Here's how the part is built. I have some questions about the finished solid (model axes, mm). A direction names the side the tool comes from. Round coordinates to 2 decimals unless told otherwise and drop trailing zeros. Write each loop counter-clockwise with the first axis right and the second up, starting at its lowest first coordinate (ties: lowest second). Pieces come first, ordered by that corner, then holes. Notation, with made-up numbers: (28, 52) - (32, 52) arc R21 ccw to (32, 80) - close; hole circle Ø8 at (88.5, 49.25). An arc over 180 degrees is marked (long way). One line per question, with ' | ' between items. Start each with the question number.
(1) Imagine slicing it at C-C (x = 174). Write out the boundary of the cut face in (y, z), plus the area to 3 significant figures.
(2) Thinking about a two-plate mould opening in Z: for faces 6 (the cylindrical face through (291.49, -377.92, 15.6)), 7 (the cylindrical face through (166.93, -15.07, 37.13)), 8 (the flat face through (213, -10, 15)), which applies, pulls with the +Z half, pulls with the -Z half, needs draft (parallel to the pull), parting line crosses it, or undercut?
(3) Imagine slicing it at B-B (x = 277). Write out the boundary of the cut face in (y, z).
(4) For faces 1 (the flat face through (99, -20, 15)), 2 (the flat face through (325.858, -237, 15)), 3 (the cylindrical face through (303.045, -34.057, 14.79)), 4 (the flat face through (325.858, -390, -9)), 5 (the flat face through (99, -10, 42)), which set-ups out of +Z, -Z, +X, -X, +Y, -Y let a thin tool reach every point of the face, with its end or its side?
(5) Imagine slicing it at A-A (x = 125). Write out the boundary of the cut face in (y, z), plus the area to 3 significant figures.
(6) Imagine slicing it at D-D (y = -180.5). Write out the boundary of the cut face in (x, z), plus the area to 3 significant figures.
(7) Will these pins go through, and if not, where does the flat tip stop? pin 1 (8 mm diameter, centred on y = -4.5, z = 33, fed in from -X); pin 2 (13.5 mm diameter, centred on x = 160, z = 40, fed in from +Y); pin 3 (10.5 mm diameter, centred on y = -390, z = -17, fed in from +X); pin 4 (5 mm diameter, centred on y = -95, z = 10.5, fed in from -X).
(8) If I drill on L1, parallel to Z at x = 75, y = -16; L2, parallel to Y at x = 46, z = 30.5; L3, parallel to Y at x = 240.5, z = 4.5, over which ranges is the centre line in solid material (lowest first)?
from build123d import *

# Parameters (mm, degrees)
SKETCH1_R           = 5
BOSS_EXTRUDE1_DEPTH = 30
SKETCH2_W           = 160
SKETCH2_H           = 20
SKETCH2_H_2         = 30
BOSS_EXTRUDE2_DEPTH = 10
RIB1_REACH          = 528.102
SKETCH5_WALL_W      = 1076.564743208
SKETCH5_WALL_H      = 10
RIB17_REACH         = 528.102
SKETCH7_WALL_W      = 1076.564743208
SKETCH7_WALL_H      = 10
SKETCH8_R           = 7.5
CUT_EXTRUDE1_DEPTH  = 10
BOSS_EXTRUDE3_DEPTH = 90
CUT_EXTRUDE3_DEPTH  = 30


with BuildPart() as part:
    # Sketch1 → Boss-Extrude1 (new body)
    with BuildSketch(Plane.XY):
        with BuildLine():
            Line((-7.071067812, 7.071067812), (75.857864376, 90))
            Line((75.857864376, 90), (345.857864376, 90))
            ThreePointArc((345.857864376, 90), (402.426406871, 66.568542495), (425.857864376, 10))
            Line((425.857864376, 10), (425.857864376, -260))
            Line((425.857864376, -260), (355.857864376, -330))
            Line((355.857864376, -330), (355.857864376, -410))
            Line((355.857864376, -410), (235.857864376, -400))
            Line((235.857864376, -400), (235.857864376, -380))
            Line((235.857864376, -380), (325.857864376, -380))
            Line((325.857864376, -380), (325.857864376, -90))
            ThreePointArc((325.857864376, -90), (302.426406871, -33.431457505), (245.857864376, -10))
            Line((245.857864376, -10), (0, -10))
            ThreePointArc((0, -10), (-9.238795325, -3.826834324), (-7.071067812, 7.071067812))
        make_face()
        Circle(SKETCH1_R, mode=Mode.SUBTRACT)
    extrude(amount=BOSS_EXTRUDE1_DEPTH)

    # Sketch2 → Boss-Extrude2 (add)
    with BuildSketch(Plane.XZ.offset(10)):
        with Locations((100, 40)):
            Rectangle(SKETCH2_W, SKETCH2_H)
        with Locations((100, 15)):
            Rectangle(SKETCH2_W, SKETCH2_H_2)
        with Locations((100, -10)):
            Rectangle(SKETCH2_W, SKETCH2_H)
    extrude(amount=BOSS_EXTRUDE2_DEPTH)

    # Sketch5 wall → Rib1 (add, up to next)
    with BuildSketch(Plane(origin=(100, 0, 35), x_dir=(0, -0.894427191, 0.4472135955), z_dir=(0, 0.4472135955, 0.894427191)), mode=Mode.PRIVATE) as rib1_sk1:
        Rectangle(SKETCH5_WALL_W, SKETCH5_WALL_H)
    rib1_tool1 = extrude(rib1_sk1.sketch, amount=-RIB1_REACH, mode=Mode.PRIVATE) - part.part
    add(rib1_tool1.solids().sort_by_distance((100, 0, 35))[0])

    # Sketch7 wall → Rib17 (add, up to next)
    with BuildSketch(Plane(origin=(100, 0, -5), x_dir=(0, -0.894427191, -0.4472135955), z_dir=(0, -0.4472135955, 0.894427191)), mode=Mode.PRIVATE) as rib17_sk1:
        Rectangle(SKETCH7_WALL_W, SKETCH7_WALL_H)
    rib17_tool1 = extrude(rib17_sk1.sketch, amount=RIB17_REACH, mode=Mode.PRIVATE) - part.part
    add(rib17_tool1.solids().sort_by_distance((100, 0, -5))[0])

    # Sketch8 → Cut-Extrude1 (cut)
    with BuildSketch(Plane.XZ.offset(20)):
        with Locations((40, 40)):
            Circle(SKETCH8_R)
        with Locations((75, 40)):
            Circle(SKETCH8_R)
        with Locations((40, -10)):
            Circle(SKETCH8_R)
        with Locations((75, -10)):
            Circle(SKETCH8_R)
        with Locations((125, -10)):
            Circle(SKETCH8_R)
        with Locations((160, -10)):
            Circle(SKETCH8_R)
        with Locations((160, 40)):
            Circle(SKETCH8_R)
        with Locations((125, 40)):
            Circle(SKETCH8_R)
    extrude(amount=-CUT_EXTRUDE1_DEPTH, mode=Mode.SUBTRACT)

    # Sketch9 → Boss-Extrude3 (add)
    with BuildSketch(Plane.ZY.offset(-325.857864376)):
        with BuildLine():
            Line((-23.890872965, -394.024153256), (-16.819805153, -401.095221068))
            ThreePointArc((-16.819805153, -401.095221068), (15, -387.915026221), (46.819805153, -401.095221068))
            Line((46.819805153, -401.095221068), (53.890872965, -394.024153256))
            ThreePointArc((53.890872965, -394.024153256), (15, -377.915026221), (-23.890872965, -394.024153256))
        make_face()
    extrude(amount=BOSS_EXTRUDE3_DEPTH)

    # Sketch10 → Cut-Extrude3 (cut)
    with BuildSketch(Plane(origin=(-31.476842315, -377.722107776, 0), x_dir=(0.9965457582448797, -0.08304547985374007, 0), z_dir=(-0.08304547985374007, -0.9965457582448797, 0))):
        Polygon((374.546486812, 58.469151485), (256.226012344, 26.776259204), (256.226012344, 62.056204403), align=None)
        Polygon((374.082224106, -28.344795763), (258.075215741, 2.728419895), (258.075215741, -32.721264486), align=None)
    extrude(amount=-CUT_EXTRUDE3_DEPTH, mode=Mode.SUBTRACT)


with BuildPart() as body_2:
    # of the pieces the cut leaves, the one that is kept (cut_extrude3_keep)
    add(part.part.solids().sort_by_distance((245.857864376, -10, 0))[0])


solid = body_2.part
Check sheet entries:
1) outline: (-20, -20) - (-10, -20) - (-10, 0) - (90, 0) - (90, 30) - (-10, 30) - (-10, 50) - (-20, 50) - close | area: 3,700 mm^2
2) face 6: parting line crosses it | face 7: undercut | face 8: needs draft
3) outline: (-403.43, 0) - (-390.49, 0) arc R45 cw to (-396.11, -10.9) - (-384.25, -10.63) arc R55 ccw to (-384.25, 40.63) - (-396.11, 40.9) arc R45 cw to (-390.49, 30) - (-403.43, 30) - close; (-16.31, 0) - (90, 0) - (90, 30) - (-16.31, 30) - close
4) face 1: +Z, -Z, -X, -Y | face 2: +Z, -Z, -X | face 3: +Z, -Z | face 4: -Z, +X, +Y, -Y | face 5: +Z, +Y
5) outline: (-20, -20) - (-10, -20) - (-10, -17.5) - (-20, -17.5) - close; (-20, -2.5) - (-10, -2.5) - (-10, 0) - (90, 0) - (90, 30) - (-10, 30) - (-10, 32.5) - (-20, 32.5) - close; (-20, 47.5) - (-10, 47.5) - (-10, 50) - (-20, 50) - close | area: 3,400 mm^2
6) outline: (325.86, 0) - (425.86, 0) - (425.86, 30) - (325.86, 30) - close | area: 3,000 mm^2
7) pin 1: x = -9.83 | pin 2: through | pin 3: x = 325.86 | pin 4: x = 325.86
8) L1: -20 to -17.5, -2.5 to 32.5, 47.5 to 50 | L2: -20 to -10 | L3: -400.39 to -378.93, -10 to 90
